Drawing for the job (mm, zero at the part's lowest x, y, z). A direction names the side the tool comes from. Round coordinates to 2 decimals unless told otherwise and drop trailing zeros. Loops run counter-clockwise (first coordinate to the right, second up) from the corner with the lowest first, then second, coordinate; pieces in that order, holes last. Notation, with made-up numbers: M 23.25,81.5 L 65.25,81.5 A15 ccw 65.25,87.5 Z; hole C 0,-2.5 d9. An arc over 180 degrees is marked long. Answer in a Markdown table with one row per item.
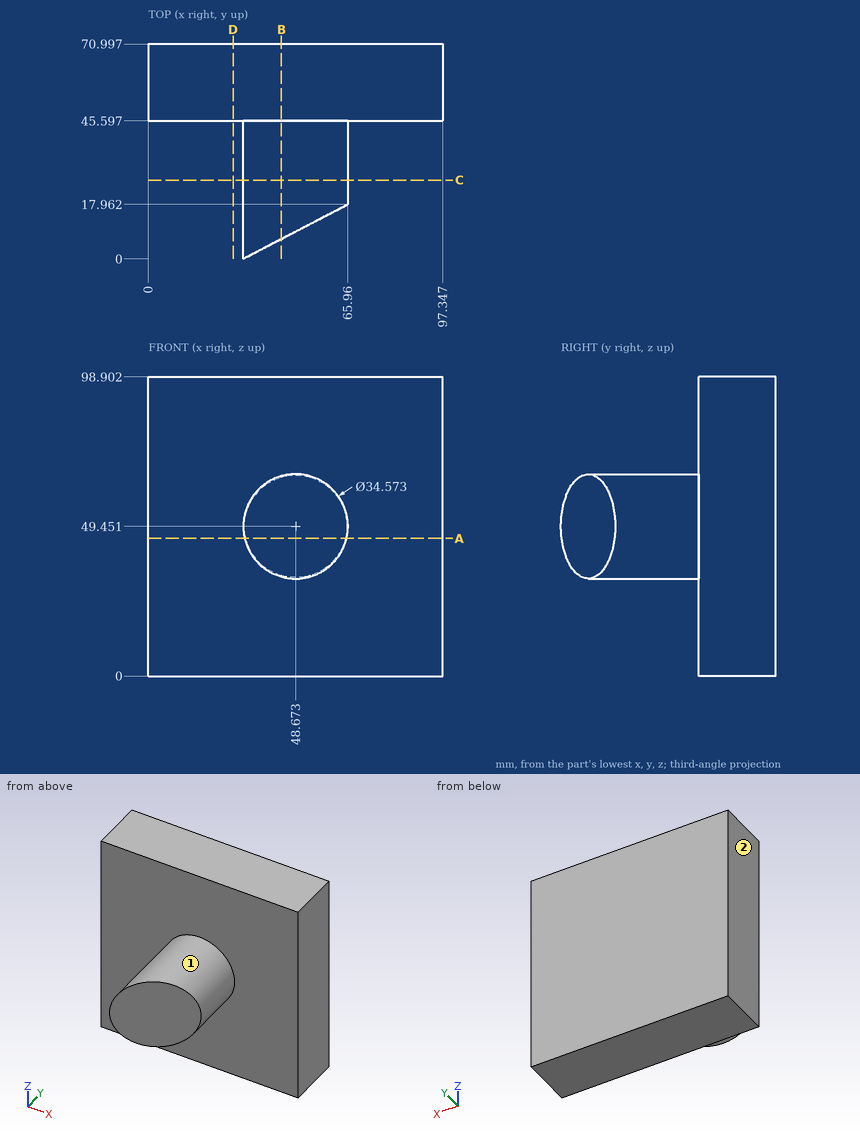
1. Pin check, flat tips, straight feed: pin 1 (10 mm diameter, centred on x = 67, z = 89, fed in from -Y); pin 2 (12 mm diameter, centred on x = 30, y = 28.5, fed in from -Z) (1 decimal); pin 3 (12 mm diameter, centred on y = 29, z = 62.5, fed in from -X). Stop position of each tip, or through.
Verdict:
| item | result |
|---|---|
| pin 1 | stops at y = 45.6 |
| pin 2 | stops at z = 37.7 |
| pin 3 | stops at x = 32.89 |
2. Saw through at C-C (y = 26). Write the cut outline in (x, z).
Verdict:
| item | result |
|---|---|
| outline | C 48.67,49.45 d34.57 |
3. Tool access for the marked faces 1 and 2: list every direction of +Z, -Z, +X, -X, +Y, -Y with a clear straight run to the whole face (end or side of a thin tool).
Verdict:
| item | result |
|---|---|
| face 1 | -Y |
| face 2 | +Z, -Z, -X, +Y, -Y |
4. Saw through at A-A (z = 45.5). Write the cut outline in (x, y) (1 decimal), and give its area (4 significant figures).
Verdict:
| item | result |
|---|---|
| outline | M 0,45.6 L 31.8,45.6 L 31.8,0.2 L 65.5,17.7 L 65.5,45.6 L 97.3,45.6 L 97.3,71 L 0,71 Z |
| area | 3,705 mm² |
5. Wall check: probe 1 along Y at (x, z) = (73, 43); probe 2 along Z at (x, y) = (39.5, 25); probe 3 along X at (y, z) = (42, 34) (1 decimal). Give the ranges that are in metal, low to high.
Verdict:
| item | result |
|---|---|
| probe 1 | y = 45.6 to 71 |
| probe 2 | z = 34.8 to 64.1 |
| probe 3 | x = 40.9 to 56.4 |
6. Saw through at D-D (x = 28). Write the cut outline in (y, z), and give its area (3 significant figures).
Verdict:
| item | result |
|---|---|
| outline | M 45.6,0 L 71,0 L 71,98.9 L 45.6,98.9 Z |
| area | 2,510 mm² |
7. Saw through at B-B (x = 44). Write the cut outline in (y, z).
Verdict:
| item | result |
|---|---|
| outline | M 6.55,32.81 L 45.6,32.81 L 45.6,0 L 71,0 L 71,98.9 L 45.6,98.9 L 45.6,66.09 L 6.55,66.09 Z |
